Read the model definition and answer for the solid it produces. Units are mm, in the model's axes. Face numbers are marked on the shaded views. A direction names the side the tool comes from. Coordinates: 2 decimals unless noted, no trailing zeros. Write each loop counter-clockwise with the first axis right and the second up, starting at its lowest first coordinate (ties: lowest second). Pieces come first, ordered by that corner, then holes.
Item 1: A tool of negligible diameter and unlimited length cuts with its end or side. For the marked faces 4, 5, 6, 7 and 8, from which of +Z, -Z, +X, -X, +Y, -Y can it reach the whole face along a straight path? Write none if from no direction.
Item 2: Section D-D (x = -16) is taken. Give the vertices of the cut face in (y, z), then the cut area to 3 significant figures.
Item 3: Section B-B (y = 7.62) is taken. Give the vertices of the cut face in (x, z) (1 decimal).
Item 4: Each of these flat-tipped pins is pushed along its axis until it touches: P1, Ø3, axis at x = -15.24, z = -6.35, coming from the +Y side; P2, Ø5.5, axis at y = 7, z = -15.5, coming from the -X side; P3, Ø0.8, axis at y = 4.5, z = -7, coming from the +X side; P4, Ø6, axis at x = -10, z = -23.5, coming from the +Y side. Where does it stop, or does it pass through?
Item 5: Straight lines are drawn through the part: probe 1 along X at (y, z) = (3, -16); probe 2 along X at (y, z) = (10, -14.5); probe 3 along X at (y, z) = (4.75, -4.5). For each, find the intervals that lie inside material, in ascending order.
Item 6: Section A-A (z = -25.4) is taken. Give the vertices of the cut face in (x, y).
Item 7: Section C-C (x = 0) is taken. Give the vertices of the cut face in (y, z) (3 decimals).
Item 8: Determine the mould class of the marked faces 1, 2 and 3 for opening direction Z: released by +Z, released by -Z, zero draft, split by the parting line, or undercut.
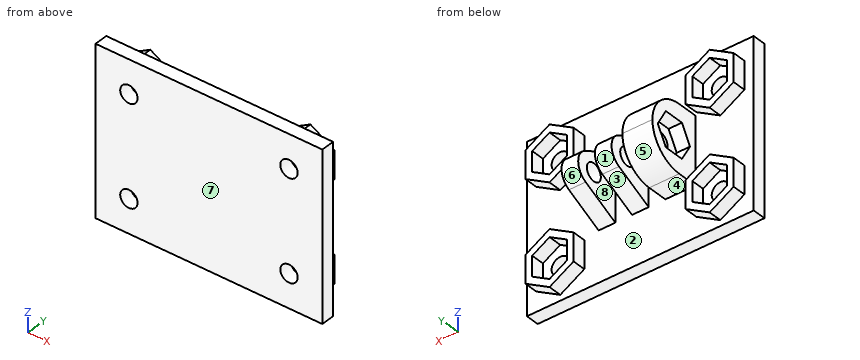
from build123d import *

# Parameters (mm, degrees)
SKETCH1_W           = 43.18
SKETCH1_H           = 31.75
SKETCH1_R           = 1.651
BOSS_EXTRUDE1_DEPTH = 2.54
SKETCH2_R           = 1.651
BOSS_EXTRUDE2_DEPTH = 7.9375
SKETCH3_W           = 3.175
SKETCH3_H           = 12.7
CUT_EXTRUDE1_DEPTH  = 12.7
FILLET1_R           = 3.175
SKETCH6_W           = 12.7
SKETCH6_H           = 10.16
SKETCH6_R           = 1.651
BOSS_EXTRUDE5_DEPTH = 3.175
SKETCH4_W           = 12.7
SKETCH4_H           = 10.16
BOSS_EXTRUDE6_DEPTH = 2.54
FILLET2_R           = 6.35
BOSS_EXTRUDE7_DEPTH = 2.54


with BuildPart() as part:
    # Sketch1 → Boss-Extrude1 (new body)
    with BuildSketch(Plane(origin=(0, 0, 0), x_dir=(1, 0, 0), z_dir=(0, 1, 0))):
        with Locations((0, 15.875)):
            Rectangle(SKETCH1_W, SKETCH1_H)
        with Locations(Location((-15.24, 25.4, 0), (0, 0, 270))):
            Circle(SKETCH1_R, mode=Mode.SUBTRACT)
        with Locations(Location((-15.24, 6.35, 0), (0, 0, 270))):
            Circle(SKETCH1_R, mode=Mode.SUBTRACT)
        with Locations(Location((15.24, 25.4, 0), (0, 0, 270))):
            Circle(SKETCH1_R, mode=Mode.SUBTRACT)
        with Locations(Location((15.24, 6.35, 0), (0, 0, 270))):
            Circle(SKETCH1_R, mode=Mode.SUBTRACT)
    extrude(amount=BOSS_EXTRUDE1_DEPTH)

    # Sketch2 → Boss-Extrude2 (add, symmetric)
    with BuildSketch(Plane(origin=(0, 0, 0), x_dir=(0, 0, -1), z_dir=(1, 0, 0))):
        Polygon((22.225, 2.54), (15.875, 15.24), (9.525, 2.54), align=None)
        with Locations((15.875, 7.62)):
            Circle(SKETCH2_R, mode=Mode.SUBTRACT)
    extrude(amount=BOSS_EXTRUDE2_DEPTH, both=True)

    # Sketch3 → Cut-Extrude1 (cut)
    with BuildSketch(Plane(origin=(0, 2.54, 0), x_dir=(1, 0, 0), z_dir=(0, 1, 0))):
        with Locations((-3.175, 15.875)):
            Rectangle(SKETCH3_W, SKETCH3_H)
        with Locations((3.175, 15.875)):
            Rectangle(SKETCH3_W, SKETCH3_H)
    extrude(amount=CUT_EXTRUDE1_DEPTH, mode=Mode.SUBTRACT)

    # Fillet1
    fillet1_edges = [part.edges().sort_by_distance(p)[0] for p in [
        (6.35, 15.24, -15.875),
        (-6.35, 15.24, -15.875),
        (0, 15.24, -15.875),
    ]]
    fillet(fillet1_edges, radius=FILLET1_R)

    # Sketch6 → Boss-Extrude5 (add)
    with BuildSketch(Plane.ZY.offset(7.9375)):
        with Locations((-15.875, 7.62)):
            Rectangle(SKETCH6_W, SKETCH6_H)
        with Locations((-15.875, 7.62)):
            Circle(SKETCH6_R, mode=Mode.SUBTRACT)
    extrude(amount=-BOSS_EXTRUDE5_DEPTH)

    # Sketch4 → Boss-Extrude6 (add)
    with BuildSketch(Plane.ZY.offset(7.9375)):
        with Locations((-15.875, 7.62)):
            Rectangle(SKETCH4_W, SKETCH4_H)
        Polygon((-19.177, 5.713589411), (-15.875, 3.807178822), (-12.573, 5.713589411), (-12.573, 9.526410589), (-15.875, 11.432821178), (-19.177, 9.526410589), align=None, mode=Mode.SUBTRACT)
    extrude(amount=BOSS_EXTRUDE6_DEPTH)

    # Fillet2
    fillet2_edges = [part.edges().sort_by_distance(p)[0] for p in [
        (-7.62, 12.7, -9.525),
        (-7.62, 12.7, -22.225),
    ]]
    fillet(fillet2_edges, radius=FILLET2_R - 0.0001)  # a hair under: the kernel refuses the full size

    # Sketch7 → Boss-Extrude7 (add)
    # profile 1 of 4: a face of its own
    with BuildSketch(Plane(origin=(0, 2.54, 0), x_dir=(1, 0, 0), z_dir=(0, 1, 0))):
        Polygon((-15.24, 30.679290861), (-19.812, 28.039645431), (-19.812, 22.760354569), (-15.24, 20.120709139), (-10.668, 22.760354569), (-10.668, 28.039645431), align=None)
        Polygon((-15.24, 29.212821178), (-18.542, 27.306410589), (-18.542, 23.493589411), (-15.24, 21.587178822), (-11.938, 23.493589411), (-11.938, 27.306410589), align=None, mode=Mode.SUBTRACT)
    # profile 2 of 4: a face of its own
    with BuildSketch(Plane(origin=(0, 2.54, 0), x_dir=(1, 0, 0), z_dir=(0, 1, 0))):
        Polygon((15.24, 30.679290861), (10.668, 28.039645431), (10.668, 22.760354569), (15.24, 20.120709139), (19.812, 22.760354569), (19.812, 28.039645431), align=None)
        Polygon((15.24, 29.212821178), (11.938, 27.306410589), (11.938, 23.493589411), (15.24, 21.587178822), (18.542, 23.493589411), (18.542, 27.306410589), align=None, mode=Mode.SUBTRACT)
    # profile 3 of 4: a face of its own
    with BuildSketch(Plane(origin=(0, 2.54, 0), x_dir=(1, 0, 0), z_dir=(0, 1, 0))):
        Polygon((15.24, 11.629290861), (10.668, 8.989645431), (10.668, 3.710354569), (15.24, 1.070709139), (19.812, 3.710354569), (19.812, 8.989645431), align=None)
        Polygon((15.24, 10.162821178), (11.938, 8.256410589), (11.938, 4.443589411), (15.24, 2.537178822), (18.542, 4.443589411), (18.542, 8.256410589), align=None, mode=Mode.SUBTRACT)
    # profile 4 of 4: a face of its own
    with BuildSketch(Plane(origin=(0, 2.54, 0), x_dir=(1, 0, 0), z_dir=(0, 1, 0))):
        Polygon((-15.24, 11.629290861), (-19.812, 8.989645431), (-19.812, 3.710354569), (-15.24, 1.070709139), (-10.668, 3.710354569), (-10.668, 8.989645431), align=None)
        Polygon((-15.24, 10.162821178), (-18.542, 8.256410589), (-18.542, 4.443589411), (-15.24, 2.537178822), (-11.938, 4.443589411), (-11.938, 8.256410589), align=None, mode=Mode.SUBTRACT)
    extrude(amount=BOSS_EXTRUDE7_DEPTH)


solid = part.part
Established:
1. face 4: -Z, +Y
1. face 5: -Z, +X, -X, +Y
1. face 6: +X, +Y
1. face 7: +Z, -Z, +X, -X, -Y
1. face 8: +Z, -Z, +Y
2. outline: (0, -31.75) - (2.54, -31.75) - (2.54, -30.24) - (5.08, -30.24) - (5.08, -28.77) - (2.54, -28.77) - (2.54, -26.87) - (0, -26.87) - close; (0, -23.93) - (2.54, -23.93) - (2.54, -22.03) - (5.08, -22.03) - (5.08, -20.56) - (2.54, -20.56) - (2.54, -11.19) - (5.08, -11.19) - (5.08, -9.72) - (2.54, -9.72) - (2.54, -7.82) - (0, -7.82) - close; (0, -4.88) - (2.54, -4.88) - (2.54, -2.98) - (5.08, -2.98) - (5.08, -1.51) - (2.54, -1.51) - (2.54, 0) - (0, 0) - close
2. area: 80.7 mm2
3. outline: (-10.5, -22.1) - (-4.8, -22.1) - (-4.8, -17.5) - (-7.9, -17.5) - (-7.9, -19.2) - (-10.5, -19.2) - close; (-10.5, -12.6) - (-7.9, -12.6) - (-7.9, -14.2) - (-4.8, -14.2) - (-4.8, -9.7) - (-10.5, -9.7) - close; (-1.6, -19.7) - (1.6, -19.7) - (1.6, -17.5) - (-1.6, -17.5) - close; (-1.6, -14.2) - (1.6, -14.2) - (1.6, -12.1) - (-1.6, -12.1) - close; (4.8, -19.7) - (7.9, -19.7) - (7.9, -17.5) - (4.8, -17.5) - close; (4.8, -14.2) - (7.9, -14.2) - (7.9, -12.1) - (4.8, -12.1) - close
4. P1: passes through
4. P2: stops at x = -10.48
4. P3: stops at x = 19.81
4. P4: stops at y = 10.7
5. probe 1: x = -10.48 to -4.76, -1.59 to 1.59, 4.76 to 7.94
5. probe 2: x = -7.94 to -4.76, -1.59 to 1.59, 4.76 to 7.94
5. probe 3: x = -19.81 to -18.54, -11.94 to -10.67, 10.67 to 11.94, 18.54 to 19.81
6. outline: (-21.59, 0) - (-16.89, 0) - (-16.89, 2.54) - (-18.54, 2.54) - (-18.54, 5.08) - (-19.81, 5.08) - (-19.81, 2.54) - (-21.59, 2.54) - close; (-13.59, 0) - (13.59, 0) - (13.59, 2.54) - (11.94, 2.54) - (11.94, 5.08) - (10.67, 5.08) - (10.67, 2.54) - (-10.67, 2.54) - (-10.67, 5.08) - (-11.94, 5.08) - (-11.94, 2.54) - (-13.59, 2.54) - close; (16.89, 0) - (21.59, 0) - (21.59, 2.54) - (19.81, 2.54) - (19.81, 5.08) - (18.54, 5.08) - (18.54, 2.54) - (16.89, 2.54) - close
7. outline: (0, -31.75) - (2.54, -31.75) - (2.54, -22.225) - (9.56, -18.715) arc R3.175 ccw to (9.56, -13.035) - (2.54, -9.525) - (2.54, 0) - (0, 0) - close; hole circle Ø3.302 at (7.62, -15.875)
8. face 1: split by the parting line
8. face 2: undercut
8. face 3: released by -Z
